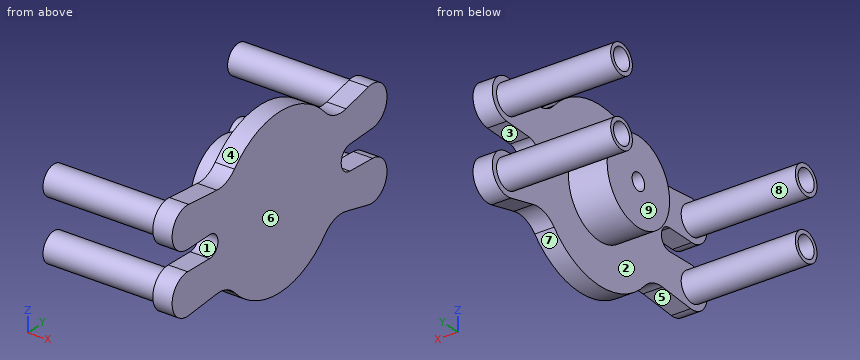
```python
from build123d import *

# Parameters (mm, degrees)
SKETCH1_W           = 17.145
SKETCH1_H           = 18.542
SKETCH2_R           = 3.71475
CUT_EXTRUDE1_DEPTH  = 8.5725
BOSS_EXTRUDE1_DEPTH = 8.5725
SKETCH4_R           = 6.44525
SKETCH4_R_2         = 4.7474251
BOSS_EXTRUDE2_DEPTH = 50.645121951


with BuildPart() as part:
    # Sketch1 → Revolve1 (revolve)
    with BuildSketch(Plane.XY):
        with Locations((16.8275, 9.271)):
            Rectangle(SKETCH1_W, SKETCH1_H)
    revolve(axis=Axis((8.255, 0, 0), (1, 0, 0)))

    # Sketch2 → Cut-Extrude1 (cut)
    with BuildSketch(Plane.ZY.offset(-8.255)):
        Circle(SKETCH2_R)
    extrude(amount=-CUT_EXTRUDE1_DEPTH, mode=Mode.SUBTRACT)

    # Sketch3 → Boss-Extrude1 (add)
    with BuildSketch(Plane(origin=(25.4, 0, 0), x_dir=(0, 0, -1), z_dir=(1, 0, 0))):
        with BuildLine():
            Line((-20.702899344, 39.448323668), (-23.827032985, 52.708168154))
            ThreePointArc((-23.827032985, 52.708168154), (-16.334994998, 63.666100226), (-6.106605949, 55.205192121))
            Line((-6.106605949, 55.205192121), (-5.453270033, 41.770518865))
            ThreePointArc((-5.453270033, 41.770518865), (0, 36.576), (5.453270033, 41.770518865))
            Line((5.453270033, 41.770518865), (6.106605949, 55.205192121))
            ThreePointArc((6.106605949, 55.205192121), (16.334994998, 63.666100226), (23.827032985, 52.708168154))
            Line((23.827032985, 52.708168154), (20.702899344, 39.448323668))
            ThreePointArc((20.702899344, 39.448323668), (20.938893682, 32.759417922), (24.542669739, 27.119386757))
            ThreePointArc((24.542669739, 27.119386757), (36.575069792, 0.260855666), (24.926987696, -26.766566093))
            ThreePointArc((24.926987696, -26.766566093), (21.721471464, -31.520323876), (20.93336456, -37.199446597))
            Line((20.93336456, -37.199446597), (22.442795242, -53.962954235))
            ThreePointArc((22.442795242, -53.962954235), (13.789101844, -63.749144471), (4.511097805, -54.552701147))
            Line((4.511097805, -54.552701147), (4.824604712, -41.518040373))
            ThreePointArc((4.824604712, -41.518040373), (0, -36.576), (-4.824604712, -41.518040373))
            Line((-4.824604712, -41.518040373), (-4.511097805, -54.552701147))
            ThreePointArc((-4.511097805, -54.552701147), (-13.789101844, -63.749144471), (-22.442795242, -53.962954235))
            Line((-22.442795242, -53.962954235), (-20.93336456, -37.199446597))
            ThreePointArc((-20.93336456, -37.199446597), (-21.721471464, -31.520323876), (-24.926987696, -26.766566093))
            ThreePointArc((-24.926987696, -26.766566093), (-36.575069792, 0.260855666), (-24.542669739, 27.119386757))
            ThreePointArc((-24.542669739, 27.119386757), (-20.938893682, 32.759417922), (-20.702899344, 39.448323668))
        make_face()
    extrude(amount=BOSS_EXTRUDE1_DEPTH)

    # Sketch4 → Boss-Extrude2 (add)
    with BuildSketch(Plane.ZY.offset(-25.4)):
        with Locations((-15.08125, 54.76875)):
            Circle(SKETCH4_R)
        with Locations((-15.08125, 54.76875)):
            Circle(SKETCH4_R_2, mode=Mode.SUBTRACT)
        with Locations((15.08125, 54.76875)):
            Circle(SKETCH4_R)
        with Locations((15.08125, 54.76875)):
            Circle(SKETCH4_R_2, mode=Mode.SUBTRACT)
        with Locations((13.49375, -54.76875)):
            Circle(SKETCH4_R)
        with Locations((13.49375, -54.76875)):
            Circle(SKETCH4_R_2, mode=Mode.SUBTRACT)
        with Locations((-13.49375, -54.76875)):
            Circle(SKETCH4_R)
        with Locations((-13.49375, -54.76875)):
            Circle(SKETCH4_R_2, mode=Mode.SUBTRACT)
    extrude(amount=BOSS_EXTRUDE2_DEPTH)


solid = part.part
```
Design review of the part built by this model. Coordinates are the model's own, in mm. Face numbers are marked on the shaded views. A direction names the side the tool comes from. Coordinates: 2 decimals unless noted, no trailing zeros. Write each loop counter-clockwise with the first axis right and the second up, starting at its lowest first coordinate (ties: lowest second). Pieces come first, ordered by that corner, then holes.
1) Add section A-A (x = -1). Write out the cut boundary in (y, z).
2) Mouldability with a two-part tool opening along Y and no side actions: class the marked faces 6, 7, 8 and 9 as +Y half, -Y half, draft (parallel to the pull), parting line (faces both ways), or undercut.
3) Machinability: for the marked faces 1, 2, 3, 4 and 5, which of the approach directions +Z, -Z, +X, -X, +Y, -Y give a long, thin tool a straight path to every point of the face, cutting with its end or side? Answer none if there is none.
4) To check wall thickness, follow L1, parallel to Y at x = 13, z = -15; L2, parallel to Y at x = -6.5, z = 16.5; L3, parallel to Y at x = -16, z = -12.5. State the ranges of each line that lie inside material, in increasing order.
5) Insertion check: pin 1 (7.5 mm diameter, centred on y = -54, z = -15, fed in from -X); pin 2 (3 mm diameter, centred on y = -55, z = 13, fed in from -X); pin 3 (22 mm diameter, centred on y = 18, z = 11, fed in from -X) (3 decimals); pin 4 (8 mm diameter, centred on x = 16, y = -17.5, fed in from -Z). Each pin has a flat end and moves straight along its axis. Give the tip position at first contact, or say it passes through.
6) Add section C-C (x = 11.5). State how many separate pieces and enclosed holes the cut face has, plus the area to 3 significant figures.
7) Add section B-B (y = 0). Write out the cut boundary in (x, z) (1 decimal), plus the area to 3 significant figures.
Check result:
1. outline: circle Ø12.89 at (-54.77, -13.49); circle Ø12.89 at (-54.77, 13.49); circle Ø12.89 at (54.77, -15.08); circle Ø12.89 at (54.77, 15.08); hole circle Ø9.49 at (-54.77, -13.49); hole circle Ø9.49 at (-54.77, 13.49); hole circle Ø9.49 at (54.77, -15.08); hole circle Ø9.49 at (54.77, 15.08)
2. face 6: draft
2. face 7: parting line
2. face 8: undercut
2. face 9: undercut
3. face 1: +X, -X
3. face 2: -X
3. face 3: +X, -X, +Y
3. face 4: +Z, +X, -X
3. face 5: -Z, +X, -X
4. L1: y = -61.04 to -59.27, -50.27 to -48.5, -10.9 to 10.9, 48.32 to 50.02, 59.52 to 61.21
4. L2: y = -60.47 to -58.44, -51.09 to -49.07, 48.48 to 50.24, 59.3 to 61.06
4. L3: y = -61.14 to -59.41, -50.13 to -48.4, 48.86 to 50.78, 58.75 to 60.67
5. pin 1: stops at x = -25.25
5. pin 2: stops at x = 25.4
5. pin 3: stops at x = 8.255
5. pin 4: stops at z = -12.71
6. separate pieces: 5
6. enclosed holes: 5
6. area: 1,280 mm2
7. outline: (8.3, -18.5) - (25.4, -18.5) - (25.4, -36.6) - (34, -36.6) - (34, 36.6) - (25.4, 36.6) - (25.4, 18.5) - (8.3, 18.5) - (8.3, 3.7) - (16.8, 3.7) - (16.8, -3.7) - (8.3, -3.7) - close
7. area: 1,200 mm2
